Geometry check sheet. Reference: drawing and pictorial views, mm from the part's lowest x, y, z. Round coordinates to 2 decimals unless told otherwise and drop trailing zeros. Order: outer loops, then holes, each group sorted by start corner. A loop starts at its lowest first (then second) coordinate and runs counter-clockwise, first axis right, second up.
(1) Depth check by flat-ended pin: pin 1 (1.6 mm diameter, centred on y = 1, z = 60, fed in from +X); pin 2 (1.6 mm diameter, centred on x = 36.5, y = 2, fed in from -Z) (1 decimal); pin 3 (1 mm diameter, centred on y = 1, z = 47, fed in from -X). Enter the tip coordinate at first touch or a pass-through.
(2) Thickness scan on probe 1 along Z at (x, y) = (34.5, 2.65) (1 decimal); probe 2 along X at (y, z) = (0.6, 26.5) (1 decimal); probe 3 along X at (y, z) = (2.9, 100) (1 decimal). Record the ranges inside material, lowest first.
(3) Sectioned sample at C-C, the plane y = 2.6. Enter the section's corners in (x, z) (1 decimal), and give its area (3 significant figures).
(4) Sectioned sample at A-A, the plane x = 6. Enter the section's corners in (y, z) (1 decimal).
(5) Sectioned sample at B-B, the plane z = 12.5. Enter the section's corners in (x, y) (1 decimal).
(6) Sectioned sample at D-D, the plane z = 46.5. Enter the section's corners in (x, y) (1 decimal).
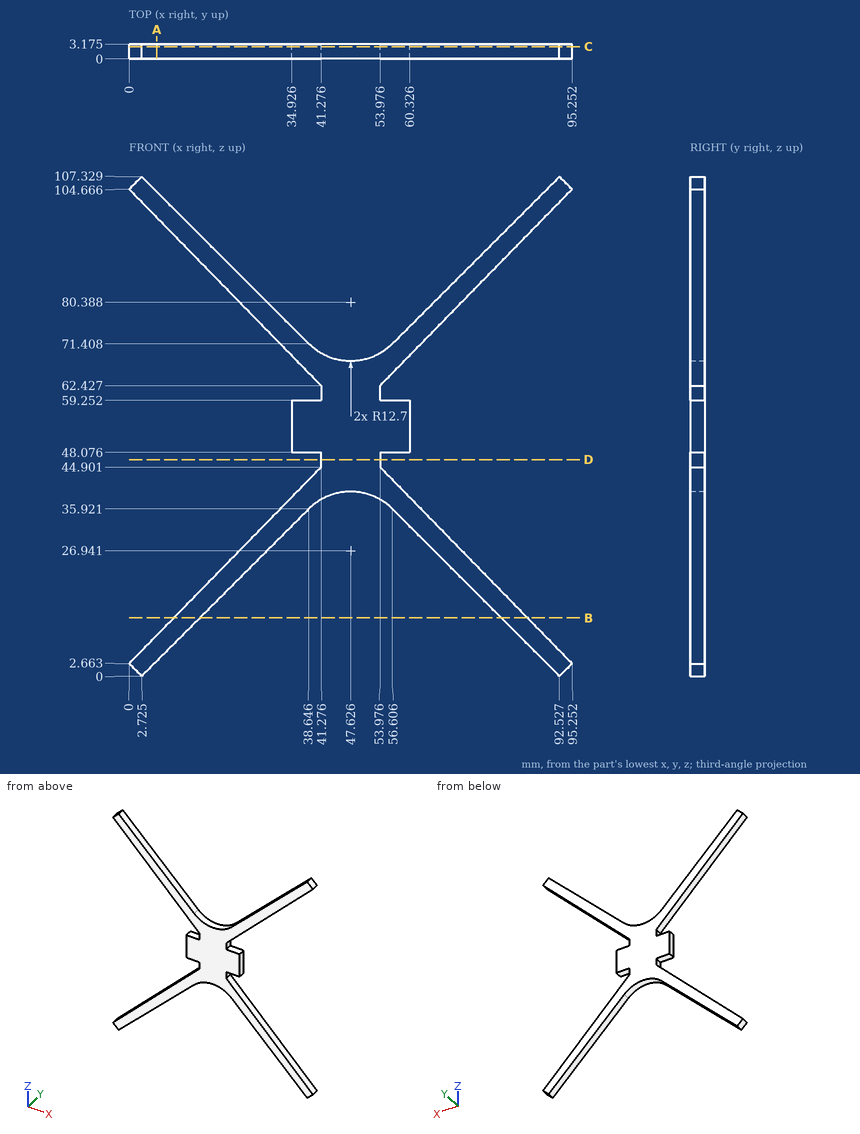
Derived:
1. pin 1: stops at x = 60.33
1. pin 2: stops at z = 33
1. pin 3: stops at x = 41.28
2. probe 1: z = 31.8 to 38, 69.4 to 75.6
2. probe 2: x = 23.3 to 29.2, 66 to 72
2. probe 3: x = 4.6 to 10.1, 85.2 to 90.7
3. outline: (0, 2.7) - (2.7, 0) - (38.6, 35.9) arc R12.7 cw to (56.6, 35.9) - (92.5, 0) - (95.3, 2.7) - (54, 44.9) - (54, 48.1) - (60.3, 48.1) - (60.3, 59.3) - (54, 59.3) - (54, 62.4) - (95.3, 104.7) - (92.5, 107.3) - (56.6, 71.4) arc R12.7 cw to (38.6, 71.4) - (2.7, 107.3) - (0, 104.7) - (41.3, 62.4) - (41.3, 59.3) - (34.9, 59.3) - (34.9, 48.1) - (41.3, 48.1) - (41.3, 44.9) - close
3. area: 1,450 mm2
4. outline: (0, 3.3) - (3.2, 3.3) - (3.2, 8.8) - (0, 8.8) - close; (0, 98.5) - (3.2, 98.5) - (3.2, 104.1) - (0, 104.1) - close
5. outline: (9.6, 0) - (15.2, 0) - (15.2, 3.2) - (9.6, 3.2) - close; (80, 0) - (85.6, 0) - (85.6, 3.2) - (80, 3.2) - close
6. outline: (41.3, 0) - (54, 0) - (54, 3.2) - (41.3, 3.2) - close
